Input: part model. Units: mm. Frame: model coordinates. A direction names the side the tool comes from. Coordinates: 2 decimals unless noted, no trailing zeros. Order: outer loops, then holes, each group sorted by start corner. A loop starts at its lowest first (then second) coordinate and runs counter-clockwise, first axis right, second up. Notation, with made-up numbers: (53.25, 48.5) - (85.25, 48.5) arc R16 cw to (85.25, 64.5) - close; hole circle Ø2 at (-5, 5). An arc over 180 degrees is marked (long way). One line per question, with ' | ' between items.
from build123d import *

# Parameters (mm, degrees)
F1_DEPTH = 25
F3_START = -7
F3_DEPTH = 4
F4_W     = 4
F4_H     = 1


with BuildPart() as f1:
    # F0 (on Top) → F1 (new body)
    with BuildSketch(Plane.XY):
        with BuildLine():
            Line((-7, -25), (7, -25))
            ThreePointArc((7, -25), (8.4142135624, -24.4142135624), (9, -23))
            Line((9, -23), (9, 23))
            ThreePointArc((9, 23), (8.4142135624, 24.4142135624), (7, 25))
            Line((7, 25), (-7, 25))
            ThreePointArc((-7, 25), (-8.4142135624, 24.4142135624), (-9, 23))
            Line((-9, 23), (-9, -23))
            ThreePointArc((-9, -23), (-8.4142135624, -24.4142135624), (-7, -25))
        make_face()
    extrude(amount=F1_DEPTH)

    # F2 (on face) → F3 (join)
    with BuildSketch(Plane.YZ.offset(9).offset(F3_START)):
        Polygon((34.6765182912, 49.9050952494), (-15.9586127847, 25), (-11.2994632265, 25), (35.5840993399, 48.0598710132), align=None)
    extrude(amount=-F3_DEPTH)

    # F4 (on face) → F5 (revolve)
    with BuildSketch(Plane(origin=(0, 47.6862617378, 23.4546818668), x_dir=(-1, 0, 0), z_dir=(0, 0.8973319166, 0.4413563543))):
        with Locations((0, 28.976733073)):
            Rectangle(F4_W, F4_H)
        Polygon((2, 28.476733073), (25, 28.476733073), (25, 30.476733073), (-25, 30.476733073), (-25, 28.476733073), (-2, 28.476733073), (-2, 29.476733073), (2, 29.476733073), align=None)
    revolve(axis=Axis((0, 35.1178746456, 49.0077633328), (1, 0, 0)))


solid = f1.part
Item 1: Section B-B on x = -8. Return the cut outline in (y, z), and give its area (3 significant figures).
Data:
outline: (-24.73, 0) - (24.73, 0) - (24.73, 25) - (-24.73, 25) - close; circle Ø4 at (35.12, 49.01) | area: 1,250 mm^2
Item 2: Section A-A on y = 2. Return the cut outline in (x, z), and give its area (3 significant figures).
Data:
outline: (-9, 0) - (9, 0) - (9, 25) - (-9, 25) - close; (-2, 31.54) - (2, 31.54) - (2, 33.83) - (-2, 33.83) - close | area: 459 mm^2
Item 3: Ray query, line 1 (X direction, y = -2.5, z = 5); line 2 (Y direction, x = -1, z = 17); line 3 (Z direction, x = 8, y = -4.5). Return the intervals inside material, ascending.
Data:
line 1: -9 to 9 | line 2: -25 to 25 | line 3: 0 to 25
Item 4: Access query for faces 1 (the face through (0, 25, 12)), 2 (the face through (8.4, -24.43, 12.32)). Directions: +Z, -Z, +X, -X, +Y, -Y. A direction counts if a zero-diameter tool reaches every point of the face in a straight line with its end or side. Return the directions, or none.
Data:
face 1: -Z, +X, -X, +Y | face 2: +Z, -Z, +X, -Y
Item 5: Section D-D on x = 20.5. Return the cut outline in (y, z), and give its area (3 significant figures).
Data:
outline: circle Ø4 at (35.12, 49.01) | area: 12.6 mm^2
Item 6: Section C-C on z = 5. Return the cut outline in (x, y).
Data:
outline: (-9, -23) arc R2 ccw to (-7, -25) - (7, -25) arc R2 ccw to (9, -23) - (9, 23) arc R2 ccw to (7, 25) - (-7, 25) arc R2 ccw to (-9, 23) - close
Item 7: Contact query for flat-ended pins moving along their axis: P1, Ø5, axis at y = -9, z = 19.5, coming from the -X side; P2, Ø12, axis at x = 3.5, y = -2.5, coming from the -Z side; P3, Ø20, axis at y = -0.5, z = 17.5, coming from the +X side; P4, Ø12, axis at y = 12, z = 39.5, coming from the +X side. Output: stop coordinate, or through.
Data:
P1: x = -9 | P2: z = 0 | P3: x = 9 | P4: x = 2
